```python
from build123d import *

# Parameters (mm, degrees)
F1_DEPTH = 10
F2_DEPTH = 12
F4_DEPTH = 10


# Not quite as in the source:
# - ends of sketch curves that miss each other by under 0.0002 mm in the source are joined


with BuildPart() as f1:
    # F0 (on Front) → F1 (new body)
    with BuildSketch(Plane.XZ):
        Polygon((0, 2), (0, 0), (64.2, 0), (64.2, 2), (62.2, 2), (2, 2), align=None)
        with BuildLine():
            Line((0, 17.5), (0, 2))
            Line((0, 2), (2, 2))
            Line((2, 2), (2, 12.5))
            ThreePointArc((2, 12.5), (3.0649650296, 13.8955071669), (4.5, 14.9065785791))
            Line((4.5, 14.9065785791), (4.5, 16.7855147476))
            Line((4.5, 16.7855147476), (2.5, 17.5))
            Line((2.5, 17.5), (0, 17.5))
        make_face()
        with BuildLine():
            Line((62.2, 2), (64.2, 2))
            Line((64.2, 2), (64.2, 17.5))
            Line((64.2, 17.5), (61.7, 17.5))
            Line((61.7, 17.5), (59.7, 16.7855148221))
            Line((59.7, 16.7855148221), (59.7, 14.9065787654))
            ThreePointArc((59.7, 14.9065787654), (61.1350349704, 13.8955073531), (62.2, 12.5000001863))
            Line((62.2, 12.5000001863), (62.2, 2))
        make_face()
    extrude(amount=F1_DEPTH)

    # F0 (on Front) → F2 (join)
    with BuildSketch(Plane.XZ):
        Polygon((0, 2), (0, 0), (64.2, 0), (64.2, 2), (62.2, 2), (2, 2), align=None)
    extrude(amount=-F2_DEPTH)

    # F3 (on face) → F4 (join)
    with BuildSketch(Plane(origin=(0, 12, 0), x_dir=(-1, 0, 0), z_dir=(0, 1, 0))):
        with BuildLine():
            Line((-64.2, 2), (-54.2, 2))
            ThreePointArc((-54.2, 2), (-59.0968473433, 3.8042035422), (-62.2, 8))
            Line((-62.2, 8), (-62.2, 10))
            Line((-62.2, 10), (-64.2, 10))
            Line((-64.2, 10), (-64.2, 2))
        make_face()
        with BuildLine():
            Line((-10, 2), (0, 2))
            Line((0, 2), (0, 10))
            Line((0, 10), (-2, 10))
            Line((-2, 10), (-2, 8))
            ThreePointArc((-2, 8), (-5.1031526567, 3.8042035422), (-10, 2))
        make_face()
    extrude(amount=-F4_DEPTH)


solid = f1.part
```
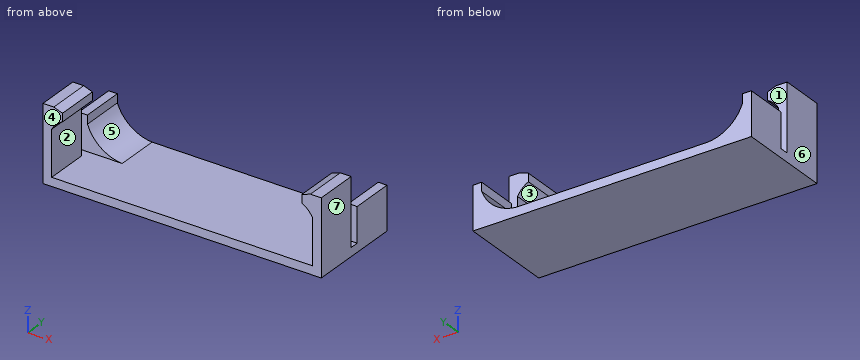
Build history of the part. All positions in model axes, mm. Face numbers are marked on the shaded views. A direction names the side the tool comes from. Give positions to 0.01 mm unless a question says otherwise; leave off trailing zeros. Order: outer loops, then holes, each group sorted by start corner. A loop starts at its lowest first (then second) coordinate and runs counter-clockwise, first axis right, second up. Notation, with made-up numbers: M -0.75,-17 L 44.25,-17 A24 ccw 44.25,21 Z; hole C 80,-26.75 d4. An arc over 180 degrees is marked long. Write item = value, one per line. Start each with the question number.
(1) Slice it at C-C on z = 4.75. Write the cut outline in (x, y), plus the area to 3 significant figures.
(2) Slice it at A-A on z = 10.75. Write the cut outline in (x, y), plus the area to 3 significant figures.
(3) Pin check, flat tips, straight feed: pin 1 Ø11 at (x, y) = (42, -2.5) entering from +Z; pin 2 Ø2 at (x, y) = (63.5, 7.5) entering from +Z. Stop position of each tip, or through.
(4) Slice it at D-D on x = 36. Write the cut outline in (y, z).
(5) Which spindle directions (+Z, -Z, +X, -X, +Y, -Y) get a long thin tool onto all of the face, cutting with end or side? Do the marked faces 1, 2 and 3. Say none if no direction does.
(6) Probe L1, parallel to X at y = -1.5, z = 4.5; L2, parallel to X at y = -2.25, z = 16.5; L3, parallel to Z at x = 50, y = 0. List the from-to ranges inside material, lowest first. Write a range as [from, to].
(7) Slice it at B-B on y = 3.75. Write the cut outline in (x, z).
(8) Two-plate mould, pull along X, no slides. Class the marked faces 4, 5, 6 and 7: released by +X, released by -X, zero draft, split by the parting line, or undercut.
Responses:
q1.outline = M 0,-10 L 2,-10 L 2,0 L 0,0 Z; M 0,2 L 4.03,2 L 4.03,12 L 0,12 Z; M 60.17,2 L 64.2,2 L 64.2,12 L 60.17,12 Z; M 62.2,-10 L 64.2,-10 L 64.2,0 L 62.2,0 Z
q1.area = 121 mm2
q2.outline = M 0,-10 L 2,-10 L 2,0 L 0,0 Z; M 62.2,-10 L 64.2,-10 L 64.2,0 L 62.2,0 Z
q2.area = 40.0 mm2
q3.pin_1 = 2
q3.pin_2 = 10
q4.outline = M -10,0 L 12,0 L 12,2 L -10,2 Z
q5.face_1 = +Z, +X, -X
q5.face_2 = -Y
q5.face_3 = +Y, -Y
q6.L1 = [0, 2], [62.2, 64.2]
q6.L2 = [0, 4.5], [59.7, 64.2]
q6.L3 = [0, 2]
q7.outline = M 0,0 L 64.2,0 L 64.2,10 L 62.2,10 L 62.2,8 A9.11 cw 54.2,2 L 10,2 A9.11 cw 2,8 L 2,10 L 0,10 Z
q8.face_4 = zero draft
q8.face_5 = undercut
q8.face_6 = released by -X
q8.face_7 = released by +X
